Geometry check sheet. Reference: the model listing, model coordinates, mm. Face numbers are marked on the shaded views. A direction names the side the tool comes from. Give positions to 0.01 mm unless a question says otherwise; leave off trailing zeros. Write each loop counter-clockwise with the first axis right and the second up, starting at its lowest first coordinate (ties: lowest second). Pieces come first, ordered by that corner, then holes. Notation, with made-up numbers: M 87,49 L 99,49 A14 cw 99,74 Z; hole C -32,-1.5 d4. An arc over 180 degrees is marked long. Write each question's results on one line, items separated by ' | '.
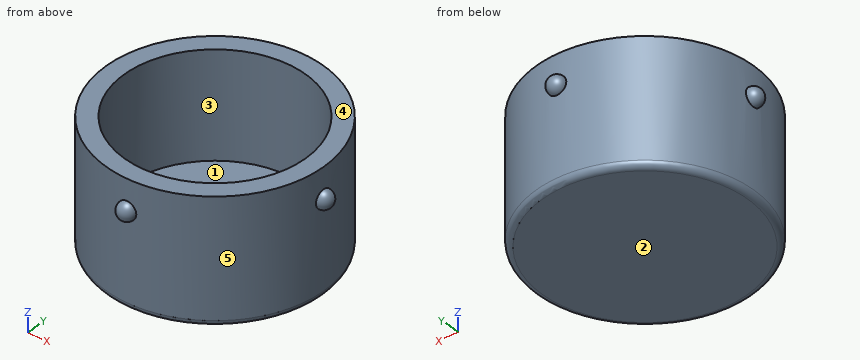
```python
from build123d import *

# Parameters (mm, degrees)
F0_R     = 36
F1_DEPTH = 41
F2_R     = 30
F3_DEPTH = 35
F7_COUNT = 4
F8_R     = 2


with BuildPart() as f1:
    # F0 (on Top) → F1 (new body)
    with BuildSketch(Plane.XY):
        Circle(F0_R)
    extrude(amount=F1_DEPTH)

    # F2 (on face) → F3 (cut)
    with BuildSketch(Plane.XY.offset(41)):
        Circle(F2_R)
    extrude(amount=-F3_DEPTH, mode=Mode.SUBTRACT)

    # F5 (on offset) → F6 (revolve)
    with BuildSketch(Plane.YZ.offset(36)):
        with BuildLine():
            Line((0, 31), (0, 28))
            ThreePointArc((0, 28), (3, 31), (0, 34))
            Line((0, 34), (0, 31))
        make_face()
    revolve(axis=Axis((36, 0, 29.6323467046), (0, 0, -1)))

    # F7: F1 ×4 about axis
    f7_axis = Axis((0, 0, 41), (0, 0, -1))


with BuildPart() as f1_1:
    add(f1.part)
    for i in range(1, F7_COUNT):
        add(f1.part.rotate(f7_axis, i * 360 / F7_COUNT))

    # F8
    f8_edges = [f1_1.edges().sort_by_distance(p)[0] for p in [
        (-36, 0, 0),
    ]]
    fillet(f8_edges, radius=F8_R)


solid = f1_1.part
```
Q1. Depth check by flat-ended pin: P1, Ø12, axis at x = -14.5, z = 24, coming from the +Y side; P2, Ø3, axis at x = 4.5, y = 25, coming from the +Z side; P3, Ø3, axis at x = -16.5, z = 27.5, coming from the +Y side. Enter the tip coordinate at first touch or a pass-through.
Answer key:
P1: stops at y = 34.98 | P2: stops at z = 6 | P3: stops at y = 32.73
Q2. Release check for a two-part mould opening along X. For the marked faces 3, 4 and 5 record: released by +X, released by -X, zero draft, split by the parting line, or undercut.
Answer key:
face 3: undercut | face 4: zero draft | face 5: split by the parting line
Q3. Section check A-A (y = 0). Enter the section's corners in (x, z).
Answer key:
outline: M -36,2 A2 ccw -34,0 L 34,0 A2 ccw 36,2 L 36,28 A3 ccw 36,34 L 36,41 L 30,41 L 30,6 L -30,6 L -30,41 L -36,41 L -36,34 A3 ccw -36,28 Z
Q4. Section check B-B (z = 30.5). Enter the section's corners in (x, y).
Answer key:
outline: M -35.88,-2.96 A36 ccw -2.96,-35.88 A2.96 ccw long 2.96,-35.88 A36 ccw 35.88,-2.96 A2.96 ccw long 35.88,2.96 A36 ccw 2.96,35.88 A2.96 ccw long -2.96,35.88 A36 ccw -35.88,2.96 A2.96 ccw long Z; hole C 0,0 d60
Q5. Access from +Z, -Z, +X, -X, +Y, -Y to the whole of each face (thin tool, end or side, straight path). Record for the marked faces 1 and 2.
Answer key:
face 1: +Z | face 2: -Z, +X, -X, +Y, -Y
Q6. Section check D-D (z = 4.5). Enter the section's corners in (x, y).
Answer key:
outline: C 0,0 d72
Q7. Material ranges on probe 1 along X at (y, z) = (0, 27); probe 2 along Y at (x, z) = (1, 24.5); probe 3 along Z at (x, y) = (-22.5, -15), recorded low to high. Write a range as [from, to].
Answer key:
probe 1: x = [-36, -30], [30, 36] | probe 2: y = [-35.99, -29.98], [29.98, 35.99] | probe 3: z = [0, 6]
